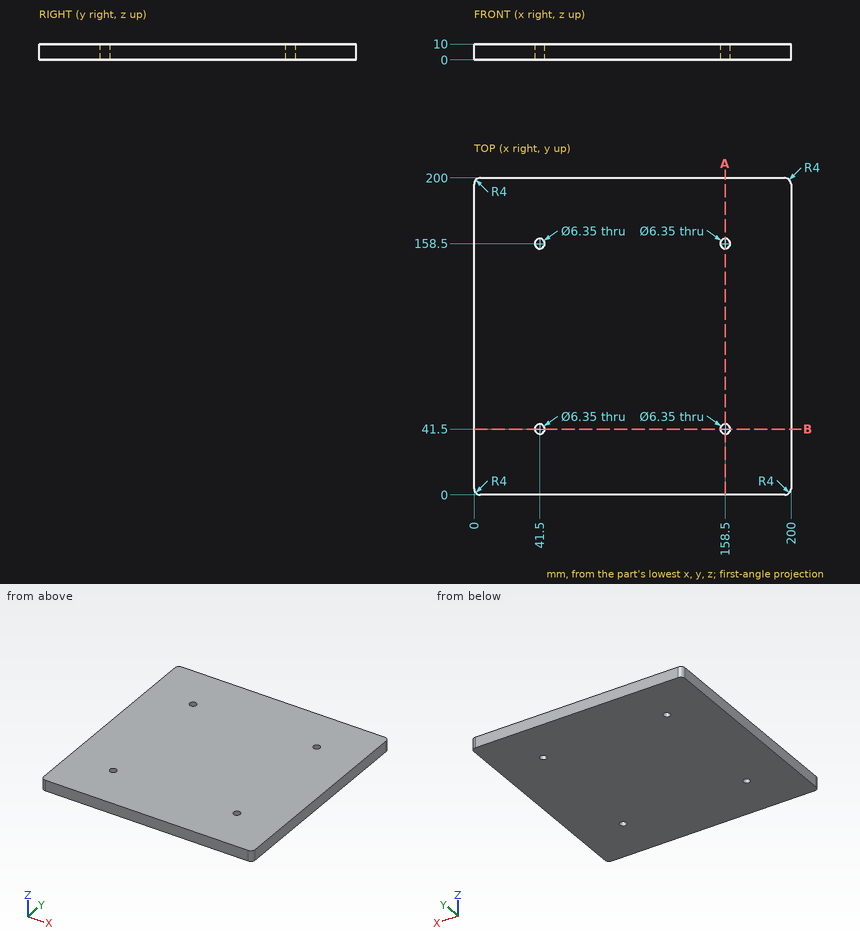
Check sheet for the drawn part. Datum: minimum x, y, z corner. Units: mm. Give positions to 0.01 mm unless a question says otherwise; leave off trailing zeros. Loops run counter-clockwise (first coordinate to the right, second up) from the corner with the lowest first, then second, coordinate; pieces in that order, holes last. Notation, with made-up numbers: (-36.75, 51) - (-11.75, 51) arc R9 cw to (-11.75, 66) - close; hole circle Ø6 at (18.5, 23). An arc over 180 degrees is marked (long way). Write each question's results on one line, items separated by ' | '.
1) Depth check by flat-ended pin: P1, Ø5, axis at x = 133.5, y = 127, coming from the -Z side. Enter the tip coordinate at first touch or a pass-through.
Solution:
P1: z = 0
2) Sectioned sample at A-A on x = 158.5. Record the boundary of the cut face in (y, z) (3 decimals), plus the area to 3 significant figures.
Solution:
outline: (0, 0) - (38.325, 0) - (38.325, 10) - (0, 10) - close; (44.675, 0) - (155.325, 0) - (155.325, 10) - (44.675, 10) - close; (161.675, 0) - (200, 0) - (200, 10) - (161.675, 10) - close | area: 1,870 mm2
3) Material ranges on L1, parallel to Y at x = 158.5, z = 6.75 (3 decimals); L2, parallel to X at y = 42, z = 8, recorded low to high. Write a range as from..to.
Solution:
L1: 0..38.325, 44.675..155.325, 161.675..200 | L2: 0..38.36, 44.64..155.36, 161.64..200
